from build123d import *

# Parameters (mm, degrees)
SKETCH1_W           = 40
SKETCH1_H           = 60
BOSS_EXTRUDE1_DEPTH = 0.8
SKETCH2_RX          = 20.672864439
SKETCH2_RY          = 20
BOSS_EXTRUDE2_DEPTH = 0.8
SKETCH5_R           = 5
SKETCH5_R_2         = 1.65
CUT_EXTRUDE3_DEPTH  = 0.8
SKETCH6_W           = 40
SKETCH6_H           = 15.577429974
CUT_EXTRUDE4_DEPTH  = 10
SKETCH7_W           = 40
SKETCH7_H           = 0.8
BOSS_EXTRUDE3_DEPTH = 10
SKETCH8_R           = 20
BOSS_EXTRUDE4_DEPTH = 0.8
SKETCH9_W           = 37.719804767
SKETCH9_H           = 12.136565496
CUT_EXTRUDE5_DEPTH  = 0.8
SKETCH10_R          = 5
SKETCH10_R_2        = 1.65
CUT_EXTRUDE8_DEPTH  = 9.8


with BuildPart() as part:
    # Sketch1 → Boss-Extrude1 (new body)
    with BuildSketch(Plane(origin=(0, 0, 0), x_dir=(1, 0, 0), z_dir=(0, 1, 0))):
        with Locations((-29.928059701, 30.852985075)):
            Rectangle(SKETCH1_W, SKETCH1_H)
    extrude(amount=BOSS_EXTRUDE1_DEPTH)

    # Sketch2 → Boss-Extrude2 (add)
    with BuildSketch(Plane(origin=(0, 0.8, 0), x_dir=(1, 0, 0), z_dir=(0, 1, 0))):
        with Locations(Location((-29.928059701, 60.852985075), (0, 0, 90))):
            Ellipse(SKETCH2_RX, SKETCH2_RY)
    extrude(amount=-BOSS_EXTRUDE2_DEPTH)

    # Sketch5 → Cut-Extrude3 (cut)
    with BuildSketch(Plane(origin=(0, 0.8, 0), x_dir=(1, 0, 0), z_dir=(0, 1, 0))):
        with Locations(Location((-30.317199226, 63.029873106, 0), (0, 0, 270))):
            Circle(SKETCH5_R)
        with Locations(Location((-30.385900954, 70.192815662, 0), (0, 0, 270))):
            Circle(SKETCH5_R_2)
        with Locations(Location((-23.205910665, 63.029873106, 0), (0, 0, 270))):
            Circle(SKETCH5_R_2)
        with Locations(Location((-37.726365539, 62.961171378, 0), (0, 0, 270))):
            Circle(SKETCH5_R_2)
        with Locations(Location((-30.454602681, 55.758110249, 0), (0, 0, 270))):
            Circle(SKETCH5_R_2)
    extrude(amount=-CUT_EXTRUDE3_DEPTH, mode=Mode.SUBTRACT)

    # Sketch6 → Cut-Extrude4 (cut)
    with BuildSketch(Plane(origin=(0, 0, 0), x_dir=(-1, 0, 0), z_dir=(0, -1, 0))):
        with Locations((29.928059701, 8.641700062)):
            Rectangle(SKETCH6_W, SKETCH6_H)
    extrude(amount=-CUT_EXTRUDE4_DEPTH, mode=Mode.SUBTRACT)

    # Sketch7 → Boss-Extrude3 (add)
    with BuildSketch(Plane(origin=(0, 0, 0), x_dir=(-1, 0, 0), z_dir=(0, -1, 0))):
        with Locations((29.928059701, 16.830415049)):
            Rectangle(SKETCH7_W, SKETCH7_H)
    extrude(amount=BOSS_EXTRUDE3_DEPTH)

    # Sketch8 → Boss-Extrude4 (add)
    with BuildSketch(Plane(origin=(0, 0, -17.230415049), x_dir=(-1, 0, 0), z_dir=(0, 0, -1))):
        with Locations((29.928059701, -10)):
            Circle(SKETCH8_R)
    extrude(amount=-BOSS_EXTRUDE4_DEPTH)

    # Sketch9 → Cut-Extrude5 (cut)
    with BuildSketch(Plane(origin=(0, 0, -17.230415049), x_dir=(-1, 0, 0), z_dir=(0, 0, -1))):
        with Locations((31.954661755, 6.868282748)):
            Rectangle(SKETCH9_W, SKETCH9_H)
    extrude(amount=-CUT_EXTRUDE5_DEPTH, mode=Mode.SUBTRACT)

    # Sketch10 → Cut-Extrude8 (cut)
    with BuildSketch(Plane(origin=(0, 0, -17.230415049), x_dir=(-1, 0, 0), z_dir=(0, 0, -1))):
        with Locations((29.816238189, -18.756032874)):
            Circle(SKETCH10_R)
        with Locations((29.853512027, -11.748551436)):
            Circle(SKETCH10_R_2)
        with Locations((37.271005677, -18.756032874)):
            Circle(SKETCH10_R_2)
        with Locations((29.816238189, -25.688966638)):
            Circle(SKETCH10_R_2)
        with Locations((22.846030588, -18.681485199)):
            Circle(SKETCH10_R_2)
    extrude(amount=-CUT_EXTRUDE8_DEPTH, mode=Mode.SUBTRACT)


solid = part.part
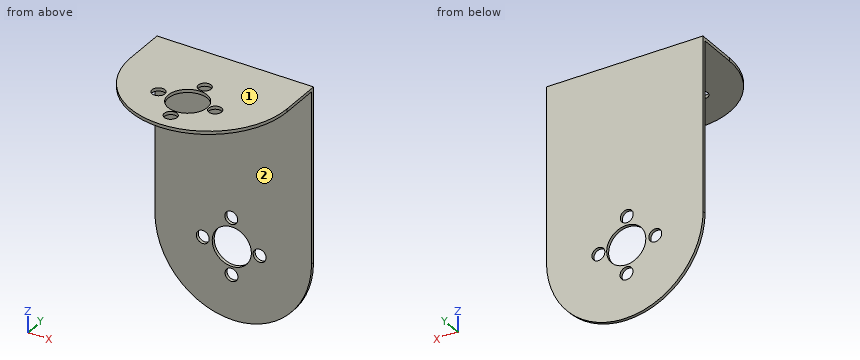
Verification items for the finished model (mm, model axes). Face numbers are marked on the shaded views. A direction names the side the tool comes from. Round coordinates to 2 decimals unless told otherwise and drop trailing zeros. Order: outer loops, then holes, each group sorted by start corner. A loop starts at its lowest first (then second) coordinate and runs counter-clockwise, first axis right, second up. Notation, with made-up numbers: (20, 3.5) -> (62, 3.5) arc R30 cw to (62, 37.5) -> close; hole circle Ø1 at (72, 32). An arc over 180 degrees is marked (long way). Put each result on its own line as item: value.
1) Set-up check for the marked faces 1 and 2: record each of +Z, -Z, +X, -X, +Y, -Y from which the full face is reachable in a straight line by a thin tool's end or side.
Final values:
face 1: +Z, +X, -X, +Y, -Y
face 2: -Z, +X, -X, -Y
2) Depth check by flat-ended pin: pin 1 (20 mm diameter, centred on x = -23.5, z = -49.5, fed in from -Y); pin 2 (2 mm diameter, centred on x = -42.5, y = -10, fed in from -Z); pin 3 (8 mm diameter, centred on x = -30.32, z = -63.03, fed in from -Y). Enter the tip coordinate at first touch or a pass-through.
Final values:
pin 1: stops at y = 0
pin 2: stops at z = -17.23
pin 3: passes through
3) Material ranges on line 1 (Y direction, x = -41, z = -26); line 2 (Z direction, x = -35, y = -23), recorded low to high.
Final values:
line 1: y = 0 to 0.8
line 2: z = -17.23 to -16.43
4) Section check A-A (y = -23). Record the cut outline in (x, z), then the cut area to 3 significant figures.
Final values:
outline: (-45.13, -17.23) -> (-32.46, -17.23) -> (-32.46, -16.43) -> (-45.13, -16.43) -> close; (-27.17, -17.23) -> (-14.73, -17.23) -> (-14.73, -16.43) -> (-27.17, -16.43) -> close
area: 20.1 mm^2
5) Section check B-B (y = -9). Record the cut outline in (x, z), then the cut area to 3 significant figures.
Final values:
outline: (-49.93, -17.23) -> (-9.93, -17.23) -> (-9.93, -16.43) -> (-49.93, -16.43) -> close
area: 32.0 mm^2
6) Section check C-C (z = -42). Record the cut outline in (x, y).
Final values:
outline: (-49.93, 0) -> (-9.93, 0) -> (-9.93, 0.8) -> (-49.93, 0.8) -> close
